Geometry check sheet. Reference: the model listing, model coordinates, mm. Round coordinates to 2 decimals unless told otherwise and drop trailing zeros. Loops run counter-clockwise (first coordinate to the right, second up) from the corner with the lowest first, then second, coordinate; pieces in that order, holes last.
```python
from build123d import *

# Parameters (mm, degrees)
BOSS_EXTRUDE1_DEPTH = 76.2
CHAMFER1_SIZE       = 16.51
CHAMFER2_SIZE       = 1
BOSS_EXTRUDE2_DEPTH = 6.35


with BuildPart() as part:
    # Sketch1 → Boss-Extrude1 (new body)
    with BuildSketch(Plane(origin=(0, 0, 0), x_dir=(1, 0, 0), z_dir=(0, 1, 0))):
        Polygon((-25.4, 47.146344636), (25.4, 47.146344636), (72.546344636, 0), (25.4, -47.146344636), (-25.4, -47.146344636), (-72.546344636, 0), align=None)
    extrude(amount=BOSS_EXTRUDE1_DEPTH)

    # SurfaceCut1
    split(bisect_by=Plane(origin=(0, 10.036699622, 10.036699622), x_dir=(-1, 0, 0), z_dir=(0, 0.7071067811865464, 0.7071067811865488)), keep=Keep.TOP)

    # SurfaceCut2
    split(bisect_by=Plane(origin=(0, 10.036699622, -10.036699622), x_dir=(1, 0, 0), z_dir=(0, 0.7071067811865464, -0.7071067811865488)), keep=Keep.TOP)

    # SurfaceCut3
    split(bisect_by=Plane(origin=(0, 50.8, 0), x_dir=(1, 0, 0), z_dir=(0, 1, 0)), keep=Keep.TOP)

    # Chamfer1
    chamfer1_edges = [part.edges().sort_by_distance(p)[0] for p in [
        (-57.183044257, 50.8, 15.363300378),
        (-57.183044257, 50.8, -15.363300378),
        (57.183044257, 50.8, 15.363300378),
        (57.183044257, 50.8, -15.363300378),
    ]]
    chamfer(chamfer1_edges, length=CHAMFER1_SIZE)

    # Chamfer2
    chamfer2_edges = [part.edges().sort_by_distance(p)[0] for p in [
        (72.546344636, 71.755, 0),
        (-72.546344636, 71.755, 0),
    ]]
    chamfer(chamfer2_edges, length=CHAMFER2_SIZE)

    # Sketch10 → Boss-Extrude2 (add)
    with BuildSketch(Plane(origin=(0, 76.2, 0), x_dir=(1, 0, 0), z_dir=(0, 1, 0))):
        Polygon((-25.4, 47.146344636), (-71.839237854, 0.707106781), (-71.839237854, -0.707106781), (-25.4, -47.146344636), (25.4, -47.146344636), (71.839237854, -0.707106781), (71.839237854, 0.707106781), (25.4, 47.146344636), align=None)
    extrude(amount=BOSS_EXTRUDE2_DEPTH)


solid = part.part
```
1) Sectioned sample at B-B, the plane z = 28. Record the cut outline in (x, y).
Report:
outline: (-44.55, 67.31) - (-21.2, 50.8) - (21.2, 50.8) - (44.55, 67.31) - (44.55, 82.55) - (-44.55, 82.55) - close
2) Scan lines: line 1 along Z through (x, y) = (-41, 75); line 2 along X through (y, z) = (74, 29); line 3 along Z through (x, y) = (-11.5, 57). Record each from-to range of solid material in increasing order.
Report:
line 1: z = -31.55 to 31.55
line 2: x = -43.55 to 43.55
line 3: z = -36.93 to 36.93
3) Sectioned sample at D-D, the plane x = -1. Record the cut outline in (y, z), then the cut area to 3 significant figures.
Report:
outline: (50.8, -30.73) - (67.22, -47.15) - (82.55, -47.15) - (82.55, 47.15) - (67.22, 47.15) - (50.8, 30.73) - close
area: 2,720 mm2
4) Sectioned sample at A-A, the plane y = 79. Record the cut outline in (x, z).
Report:
outline: (-71.84, -0.71) - (-25.4, -47.15) - (25.4, -47.15) - (71.84, -0.71) - (71.84, 0.71) - (25.4, 47.15) - (-25.4, 47.15) - (-71.84, 0.71) - close
5) Sectioned sample at C-C, the plane x = 51. Record the cut outline in (y, z), then the cut area to 3 significant figures.
Report:
outline: (52.07, 0) - (67.31, -21.55) - (82.55, -21.55) - (82.55, 21.55) - (67.31, 21.55) - close
area: 985 mm2
6) Gauge pin test, flat ends, axial feed: pin 1 (10 mm diameter, centred on y = 74.5, z = -32.5, fed in from +X); pin 2 (4 mm diameter, centred on y = 65, z = 36.5, fed in from +X); pin 3 (5 mm diameter, centred on y = 68, z = -16.5, fed in from +X). Record the tip position at first contact, or that the pin passes through.
Report:
pin 1: stops at x = 45.05
pin 2: stops at x = 36.24
pin 3: stops at x = 58.55
